from build123d import *

# Parameters (mm, degrees)
VERTICALSUPPORT_START     = -8.727944435
VERTICALSUPPORT_OUTLINE_W = 4.644211625
VERTICALSUPPORT_OUTLINE_H = 39.932212354
VERTICALSUPPORT_DEPTH     = 3.175
SKETCH1_W                 = 7.5
SKETCH1_H                 = 17.511250173
CUT_EXTRUDE1_DEPTH        = 70.171999778


# Read off the part's stored shape, not the designer's step: VerticalSupport
with BuildPart() as part:
    # VerticalSupport outline → VerticalSupport (new body)
    with BuildSketch(Plane.YZ.offset(VERTICALSUPPORT_START)):
        with BuildLine():
            Line((3.674649338, -56.776141905), (13.071575546, -60.196343338))
            Line((13.071575546, -60.196343338), (14.157489501, -57.212819267))
            Line((14.157489501, -57.212819267), (25.850623416, -61.468771968))
            add(Edge.make_bspline(
                [(24.902673716, -17.12538653), (30.294038787, -30.457344803), (31.214851934, -44.900745737), (25.850623416, -61.468771968)],
                knots=[0.580400882, 0.580400882, 0.580400882, 0.580400882, 0.976268241, 0.976268241, 0.976268241, 0.976268241], degree=3))
            Line((24.902673716, -17.12538653), (14.394673716, -14.74413653))
            Line((14.394673716, -14.74413653), (14.394673716, -17.12538653))
            Line((14.394673716, -17.12538653), (-10.888823942, -17.12538653))
            Line((-10.888823942, -17.12538653), (-10.888823942, -10.55438653))
            Line((-10.888823942, -10.55438653), (-7.713823942, -10.55438653))
            Line((-7.713823942, -10.55438653), (-7.713823942, -0.04638653))
            Line((-7.713823942, -0.04638653), (-10.888823942, -0.04638653))
            Line((-10.888823942, -0.04638653), (-10.888823942, 10.72461347))
            Line((-10.888823942, 10.72461347), (6.622426231, 10.72461347))
            add(Edge.make_bspline(
                [(-21.922009797, 37.540280116), (-11.188458316, 28.533761028), (-1.433315203, 19.729402601), (6.622426231, 10.72461347)],
                knots=[0, 0, 0, 0, 0.291032797, 0.291032797, 0.291032797, 0.291032797], degree=3))
            Line((-21.922009797, 37.540280116), (-26.742916869, 31.794946793))
            Line((-26.742916869, 31.794946793), (-24.310725762, 29.754096132))
            Line((-24.310725762, 29.754096132), (-28.388823942, 24.894007976))
            Line((-28.388823942, 24.894007976), (-28.388823942, 16.04961347))
            Line((-28.388823942, 16.04961347), (-31.563823942, 16.04961347))
            Line((-31.563823942, 16.04961347), (-31.563823942, 1.04961347))
            Line((-31.563823942, 1.04961347), (-28.388823942, 1.04961347))
            Line((-28.388823942, 1.04961347), (-28.388823942, -21.45038653))
            Line((-28.388823942, -21.45038653), (-31.563823942, -21.45038653))
            Line((-31.563823942, -21.45038653), (-31.563823942, -36.45038653))
            Line((-31.563823942, -36.45038653), (-28.388823942, -36.45038653))
            Line((-28.388823942, -36.45038653), (-28.388823942, -41.727227597))
            Line((-28.388823942, -41.727227597), (-23.430215331, -43.532013534))
            Line((-23.430215331, -43.532013534), (-24.516129286, -46.515537605))
            Line((-24.516129286, -46.515537605), (-15.119203078, -49.935739039))
            Line((-15.119203078, -49.935739039), (-14.033289123, -46.952214968))
            Line((-14.033289123, -46.952214968), (4.760563293, -53.792617834))
            Line((4.760563293, -53.792617834), (3.674649338, -56.776141905))
        make_face()
        with Locations((-20.51645306, -8.993872337)):
            Rectangle(VERTICALSUPPORT_OUTLINE_W, VERTICALSUPPORT_OUTLINE_H, mode=Mode.SUBTRACT)
    extrude(amount=VERTICALSUPPORT_DEPTH)

    # Sketch1 → Cut-Extrude1 (cut, through all)
    with BuildSketch(Plane(origin=(-5.552944435, 0, 0), x_dir=(0, 0, -1), z_dir=(1, 0, 0))):
        with Locations((-14.47461347, -2.133198855)):
            Rectangle(SKETCH1_W, SKETCH1_H)
    extrude(amount=-CUT_EXTRUDE1_DEPTH, mode=Mode.SUBTRACT)


solid = part.part
Geometry: final body of the model. Coordinates: model frame, mm. A direction names the side the tool comes from. Give positions to 0.01 mm unless a question says otherwise; leave off trailing zeros. Loops run counter-clockwise (first coordinate to the right, second up) from the corner with the lowest first, then second, coordinate; pieces in that order, holes last. Notation, with made-up numbers: (56.25, 9.5) - (92.25, 9.5) arc R15 ccw to (92.25, 15.5) - close; hole circle Ø7 at (12.5, 63). An arc over 180 degrees is marked (long way). One line per question, with ' | ' between items. Start each with the question number.
(1) Pull-direction query (Y, two-part tool) for faces 4 (the flat face through (-7, 2, -17.125)), 5 (the flat face through (-7, -9, -10.554)), 6 (the flat face through (-7, -21, -28.96)), 7 (the flat face through (-7.163, -23.966, -45.003)); classes: released by +Y, released by -Y, zero draft, split by the parting line, or undercut.
(2) Reachability of faces 1 (the flat face through (-7, -30, 1.05)), 2 (the flat face through (-7.163, 13.607, -58.725)), 3 (the flat face through (-7, -6, 18.225)) from +Z, -Z, +X, -X, +Y, -Y: full face, straight path, thin tool, end or side. Return the list, or none.
(3) Contact query for flat-ended pins moving along their axis: pin 1 (1 mm diameter, centred on x = -7.5, y = -30.5, fed in from -Z); pin 2 (1.9 mm diameter, centred on x = -6.5, z = -16.5, fed in from -Y); pin 3 (2 mm diameter, centred on y = -9, z = 8.5, fed in from -X); pin 4 (1.6 mm diameter, centred on x = -6.5, z = 13, fed in from +Y). Output: stop coordinate, or through.
(4) Section query A-A on z = -7. Return loops of the section in (x, y), then the cut area to 3 significant figures.
(5) Ray query, line 1 (Y direction, x = -6.05, z = 8); line 2 (Z direction, x = -8.2, y = -10); line 3 (Y direction, x = -7.35, z = -4). Return the intervals inside material, ascending. Write a range as from..to.
(6) Section query B-B on y = 15.5. Return loops of the section in (x, z), then the cut area to 3 significant figures.
(7) Section query C-C on y = 23. Return loops of the section in (x, z), then the cut area to 3 significant figures.
The answers:
1) face 4: undercut | face 5: zero draft | face 6: undercut | face 7: released by -Y
2) face 1: +X, -X, -Y | face 2: -Z, +X, -X | face 3: +X, -X, +Y
3) pin 1: z = -36.45 | pin 2: y = -28.39 | pin 3: through | pin 4: y = -10.89
4) outline: (-8.73, -28.39) - (-5.55, -28.39) - (-5.55, -22.84) - (-8.73, -22.84) - close; (-8.73, -18.19) - (-5.55, -18.19) - (-5.55, -7.71) - (-8.73, -7.71) - close | area: 50.9 mm2
5) line 1: -31.56..-22.84, -18.19..-10.89 | line 2: -48.42..-17.13, -10.55..-0.05, 18.22..27.2 | line 3: -28.39..-22.84, -18.19..-7.71
6) outline: (-8.73, -57.7) - (-5.55, -57.7) - (-5.55, -14.99) - (-8.73, -14.99) - close | area: 136 mm2
7) outline: (-8.73, -60.43) - (-5.55, -60.43) - (-5.55, -16.69) - (-8.73, -16.69) - close | area: 139 mm2
